Could you check a few things on this model? Use its own coordinates, in mm. A direction names the side the tool comes from. Give positions to 0.01 mm unless a question says otherwise; leave off trailing zeros. Loops run counter-clockwise (first coordinate to the right, second up) from the corner with the lowest first, then second, coordinate; pieces in that order, holes last. Notation, with made-up numbers: (-36, 21.25) -> (10, 21.25) arc R16 cw to (10, 49.25) -> close; hole circle Ø5 at (34.25, 38.25). An arc over 180 degrees is marked (long way). Write item = value, one per line. Start each with the question number.
1) I'm going to push flat-ended pins straight in: pin 1 Ø1 at (x, y) = (0, 0) entering from -Z; pin 2 Ø1 at (x, z) = (1.5, -1) entering from +Y; pin 3 Ø0.8 at (x, z) = (0, 0) entering from +Y; pin 4 Ø1.5 at (x, y) = (1.5, -2) entering from -Z. Where does each tip first touch, or does it pass through?
2) I want a section at A-A (y = 2.1). List the corners of the cut face in (x, z) for me, and give its area (3 significant figures).
3) On a 3-axis mill with a long thin cutter (end or side, diameter ignored), from which of +Z, -Z, +X, -X, +Y, -Y can I reach the whole of each face in a straight line? I mean faces 4 (the face through (0, -3, 0)), 5 (the face through (0, 1.5, 0)), 6 (the face through (0, -1, 1)). Say none if no direction works.
4) I need wall thicknesses on probe 1 along Y at (x, z) = (0, 1.3); probe 2 along Z at (x, y) = (-0.6, 2.75); probe 3 along Z at (x, y) = (-0.05, -1.6). Which ranges of each line are inside material? Lowest first, please. Write a range as from..to.
5) I want a section at D-D (y = 1.25). List the corners of the cut face in (x, z) for me, and give its area (3 significant figures).
6) If we mould it in two halves opening along Z, with no side actions, what happens to faces 1 (the face through (-1.9, 1.87, -0.08)), 2 (the face through (1, 3, 0)), 3 (the face through (0.75, 2, 0))? For each: +Z half, -Z half, draft (parallel to the pull), parting line (faces both ways), or undercut.
7) I want a section at B-B (z = 0). List the corners of the cut face in (x, y) for me, and give its area (3 significant figures).
8) I want a section at C-C (y = -0.6). List the corners of the cut face in (x, z) for me, and give its area (3 significant figures).
Autodesk Inventor part; units mm, degrees
ref_plane "YZ Plane" through (0, 0, 0) normal (1, 0, 0) x (0, 1, 0)
ref_plane "XZ Plane" through (0, 0, 0) normal (0, 1, 0) x (-1, 0, 0)
ref_plane "XY Plane" through (0, 0, 0) normal (0, 0, 1) x (1, 0, 0)
sketch "Sketch1" plane through (0, 0, 0) normal (0, 0, 1) x (1, 0, 0)
  line L0 (0, 3) -> (0, -3)
  line L1 (0, -3) -> (0.75, -3)
  line L2 (0.75, -3) -> (1, -2.75)
  line L3 (1, -2.75) -> (1, 0.75)
  line L4 (1.25, 1) -> (1.9, 1)
  line L5 (1.9, 1) -> (1.9, 2.7113)
  line L6 (1.4, 3) -> (0, 3)
  arc A0 (1.25, 1) -> (1, 0.75) centre (1.25, 0.75) ccw
  line L7 (1.4, 3) -> (1.9, 2.7113)
  point P0 (0, 0)
  point P1 (1.9, 3)
  point P2 (0, 0)
  dimension "d0" = 3.8
  dimension "d1" = 2
  dimension "d3" = 2
  dimension "d4" = 2.5
  dimension "d5" = 135
  dimension "d6" = 0.25
  dimension "d7" = 4
  dimension "d9" = 0.5
  dimension "d10" = 30
revolve "Revolution1" add sketch "Sketch1" angle 360 about axis through (0, 3, 0) along (0, -1, 0)
sketch "Sketch2" plane through (0, 3, 0) normal (0, 1, 0) x (1, 0, 0)
  line L0 (0, -0.866) -> (-0.75, -0.433)
  line L1 (-0.75, -0.433) -> (-0.75, 0.433)
  line L2 (-0.75, 0.433) -> (0, 0.866)
  line L3 (0, 0.866) -> (0.75, 0.433)
  line L4 (0.75, 0.433) -> (0.75, -0.433)
  line L5 (0.75, -0.433) -> (0, -0.866)
  point P0 (0, 0)
  point P1 (0, 0)
  dimension "d11" = 1.5
extrude "Extrusion1" cut sketch "Sketch2" against normal blind 1.5
thread "Thread1"
properties part number "Bolt_M2x0.4_4mm_SH" material "Stainless Steel"
Answer list:
q1.pin_1 = -1
q1.pin_2 = 3
q1.pin_3 = 1.5
q1.pin_4 = -0.66
q2.outline = circle Ø3.8 at (0, 0); hole (-0.75, -0.43) -> (0, -0.87) -> (0.75, -0.43) -> (0.75, 0.43) -> (0, 0.87) -> (-0.75, 0.43) -> close
q2.area = 9.39 mm^2
q3.face_4 = +Z, -Z, +X, -X, -Y
q3.face_5 = +Y
q3.face_6 = -Y
q4.probe_1 = 1..3
q4.probe_2 = -1.73..-0.52, 0.52..1.73
q4.probe_3 = -1..1
q5.outline = circle Ø3.8 at (0, 0)
q5.area = 11.3 mm^2
q6.face_1 = parting line
q6.face_2 = draft
q6.face_3 = undercut
q7.outline = (-1.9, 1) -> (-1.25, 1) arc R0.25 cw to (-1, 0.75) -> (-1, -2.75) -> (-0.75, -3) -> (0.75, -3) -> (1, -2.75) -> (1, 0.75) arc R0.25 cw to (1.25, 1) -> (1.9, 1) -> (1.9, 2.71) -> (1.4, 3) -> (0.75, 3) -> (0.75, 1.5) -> (-0.75, 1.5) -> (-0.75, 3) -> (-1.4, 3) -> (-1.9, 2.71) -> close
q7.area = 13.2 mm^2
q8.outline = circle Ø2 at (0, 0)
q8.area = 3.14 mm^2
